Verification items for the finished model (mm, model axes). Face numbers are marked on the shaded views. A direction names the side the tool comes from. Give positions to 0.01 mm unless a question says otherwise; leave off trailing zeros. Write each loop counter-clockwise with the first axis right and the second up, starting at its lowest first coordinate (ties: lowest second). Pieces come first, ordered by that corner, then holes. Notation, with made-up numbers: M 46,17.5 L 104,17.5 A4 cw 104,22.5 Z; hole C 6.5,-8 d11. An arc over 180 degrees is marked long. Write item = value, one per line.
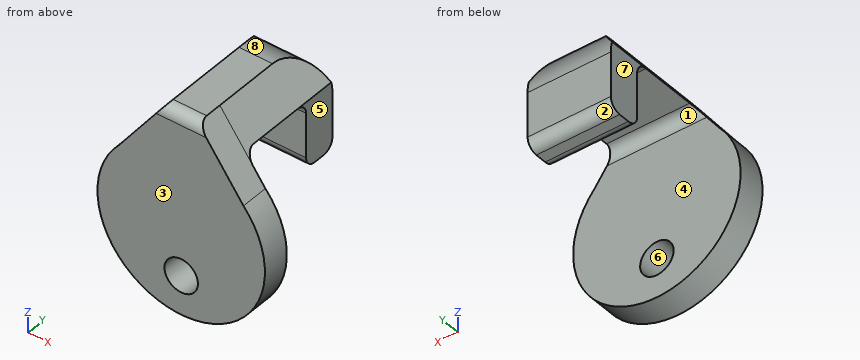
from build123d import *

# Parameters (mm, degrees)
SKETCH1_R           = 3
BOSS_EXTRUDE2_DEPTH = 5
SKETCH2_W           = 6
SKETCH2_H           = 6
BOSS_EXTRUDE5_DEPTH = 20
SKETCH6_W           = 14.919898766
SKETCH6_H           = 6
BOSS_EXTRUDE6_DEPTH = 12
FILLET2_R           = 8
FILLET3_R           = 2
FILLET4_R           = 2
FILLET5_R           = 2
FILLET6_R           = 2


with BuildPart() as part:
    # Sketch1 → Boss-Extrude2 (new body)
    with BuildSketch(Plane(origin=(0, 0, 0), x_dir=(1, 0, 0), z_dir=(0, 1, 0))):
        with BuildLine():
            ThreePointArc((11.158287634, -10.024600595), (0, 15), (-11.158287634, -10.024600595))
            Line((-11.158287634, -10.024600595), (-3, -21))
            Line((-3, -21), (3, -21))
            Line((3, -21), (11.158287634, -10.024600595))
        make_face()
        with Locations(Location((0, 8, 0), (0, 0, 270))):
            Circle(SKETCH1_R, mode=Mode.SUBTRACT)
    extrude(amount=BOSS_EXTRUDE2_DEPTH)

    # Sketch2 → Boss-Extrude5 (add)
    with BuildSketch(Plane(origin=(0, 5, 0), x_dir=(1, 0, 0), z_dir=(0, 1, 0))):
        Polygon((-7.459949383, -15), (-3, -21), (-3, -15), align=None)
        with Locations((0, -18)):
            Rectangle(SKETCH2_W, SKETCH2_H)
        Polygon((3, -15), (3, -21), (7.459949383, -15), align=None)
    extrude(amount=BOSS_EXTRUDE5_DEPTH)

    # Sketch6 → Boss-Extrude6 (add)
    with BuildSketch(Plane(origin=(0, 0, 15), x_dir=(-1, 0, 0), z_dir=(0, 0, -1))):
        with Locations((0, 22)):
            Rectangle(SKETCH6_W, SKETCH6_H)
    extrude(amount=BOSS_EXTRUDE6_DEPTH)

    # Fillet2
    fillet2_edges = [part.edges().sort_by_distance(p)[0] for p in [
        (0, 25, 21),
    ]]
    fillet(fillet2_edges, radius=FILLET2_R)

    # Fillet3
    fillet3_edges = [part.edges().sort_by_distance(p)[0] for p in [
        (0, 5, 15),
    ]]
    fillet(fillet3_edges, radius=FILLET3_R)

    # Fillet4
    fillet4_edges = [part.edges().sort_by_distance(p)[0] for p in [
        (0, 19, 15),
    ]]
    fillet(fillet4_edges, radius=FILLET4_R)

    # Fillet5
    fillet5_edges = [part.edges().sort_by_distance(p)[0] for p in [
        (0, 0, 21),
    ]]
    fillet(fillet5_edges, radius=FILLET5_R)

    # Fillet6
    fillet6_edges = [part.edges().sort_by_distance(p)[0] for p in [
        (0, 19, 3),
        (0, 25, 3),
    ]]
    fillet(fillet6_edges, radius=FILLET6_R)


solid = part.part
1) Cross-section at D-D on y = 16. Record the boundary of the cut face in (x, z), plus the area to 3 significant figures.
From the geometry:
outline = M -7.46,15 L 7.46,15 L 3,21 L -3,21 Z
area = 62.8 mm^2
2) Draft check along Y on the marked faces 1, 2 and 3. Enter one of: +Y half, -Y half, draft (parallel to the pull), parting line (faces both ways), or undercut.
From the geometry:
face_1 = undercut
face_2 = +Y half
face_3 = -Y half
3) Material ranges on probe 1 along Y at (x, z) = (-5, 10); probe 2 along Z at (x, y) = (-1.5, 11.75); probe 3 along Y at (x, z) = (0, 4.5), recorded low to high. Write a range as from..to.
From the geometry:
probe_1 = 0..5, 19..25
probe_2 = 15..21
probe_3 = 0..5, 19.06..24.94
4) Depth check by flat-ended pin: P1, Ø6.5, axis at x = -3.5, z = 9.5, coming from the -Y side; P2, Ø1.5, axis at y = 12, z = 15, coming from the -X side; P3, Ø12, axis at x = -9.5, y = 7, coming from the +Z side; P4, Ø1.6, axis at x = 1.5, y = 21.5, coming from the -Z side. Enter the tip coordinate at first touch or a pass-through.
From the geometry:
P1 = 0
P2 = -7.46
P3 = 20.33
P4 = 3
5) Cross-section at A-A on x = 0. Record the boundary of the cut face in (y, z).
From the geometry:
outline = M 0,-15 L 5,-15 L 5,-11 L 0,-11 Z; M 0,-5 L 5,-5 L 5,13 A2 cw 7,15 L 17,15 A2 cw 19,13 L 19,5 A2 ccw 21,3 L 23,3 A2 ccw 25,5 L 25,13 A8 ccw 17,21 L 2,21 A2 ccw 0,19 Z
6) Cross-section at B-B on z = -8. Record the boundary of the cut face in (x, y), plus the area to 3 significant figures.
From the geometry:
outline = M -12.69,0 L -3,0 L -3,5 L -12.69,5 Z; M 3,0 L 12.69,0 L 12.69,5 L 3,5 Z
area = 96.9 mm^2
7) Cross-section at C-C on x = 6. Record the boundary of the cut face in (y, z), plus the area to 3 significant figures.
From the geometry:
outline = M 0,-13.75 L 5,-13.75 L 5,13 A2 cw 7,15 L 17,15 A2 cw 19,13 L 19,5 A2 ccw 21,3 L 23,3 A2 ccw 25,5 L 25,13 A8 ccw 23.95,16.96 L 0,16.96 Z
area = 263 mm^2
8) Tool access check on the marked faces 4, 5, 6, 7 and 8. Record the directions out of +Z, -Z, +X, -X, +Y, -Y that give a thin tool (end or side, any length) a straight path to the whole face; none if there is none.
From the geometry:
face_4 = -Z, +X, -X
face_5 = +Z, -Z, +X, +Y
face_6 = +Y, -Y
face_7 = +Z, -Z, -X, +Y
face_8 = +Z, +X, -X, +Y
